Work out the finished part from the listing and answer in its coordinate system (mm). A direction names the side the tool comes from. Give positions to 0.01 mm unless a question says otherwise; leave off trailing zeros. Order: outer loops, then holes, each group sorted by start corner. A loop starts at its lowest first (then second) coordinate and runs counter-clockwise, first axis right, second up.
```python
from build123d import *

# Parameters (mm, degrees)
ESQUISSE1_R             = 75
ESQUISSE1_R_2           = 70
ESQUISSE1_R_3           = 2
ESQUISSE1_W             = 21
ESQUISSE1_H             = 41
BOSS_EXTRU_1_DEPTH      = 2
BOSS_EXTRU_2_START      = 40
ESQUISSE1_4_R           = 75
ESQUISSE1_4_R_2         = 70
BOSS_EXTRU_2_DEPTH      = 40
ESQUISSE2_W             = 20.133446777
ESQUISSE2_H             = 7.336961674
ENL_V_MAT_EXTRU_1_DEPTH = 40
ESQUISSE1_5_R           = 75
ESQUISSE1_5_R_2         = 70
BOSS_EXTRU_3_DEPTH      = 18


with BuildPart() as part:
    # Esquisse1 → Boss.-Extru.1 (new body)
    # profile 1 of 2: a face of its own
    with BuildSketch(Plane(origin=(0, 0, 0), x_dir=(1, 0, 0), z_dir=(0, 1, 0))):
        with Locations(Location((0, 0, 0), (0, 0, 270))):
            Circle(ESQUISSE1_R)
        Circle(ESQUISSE1_R_2, mode=Mode.SUBTRACT)
    # profile 2 of 2: a face of its own
    with BuildSketch(Plane(origin=(0, 0, 0), x_dir=(1, 0, 0), z_dir=(0, 1, 0))):
        Circle(ESQUISSE1_R_2)
        with Locations(Location((5, 14.17927264, 0), (0, 0, 270))):
            Circle(ESQUISSE1_R_3, mode=Mode.SUBTRACT)
        with Locations(Location((-5, 14.17927264, 0), (0, 0, 270))):
            Circle(ESQUISSE1_R_3, mode=Mode.SUBTRACT)
        with Locations(Location((-5, -34.45072736, 0), (0, 0, 270))):
            Circle(ESQUISSE1_R_3, mode=Mode.SUBTRACT)
        with Locations(Location((5, -34.45072736, 0), (0, 0, 270))):
            Circle(ESQUISSE1_R_3, mode=Mode.SUBTRACT)
        with Locations((0, -10.2)):
            Rectangle(ESQUISSE1_W, ESQUISSE1_H, mode=Mode.SUBTRACT)
    extrude(amount=-BOSS_EXTRU_1_DEPTH)

    # Esquisse1_4 → Boss.-Extru.2 (add)
    with BuildSketch(Plane(origin=(0, 0, 0), x_dir=(1, 0, 0), z_dir=(0, 1, 0)).offset(BOSS_EXTRU_2_START)):
        with Locations(Location((0, 0, 0), (0, 0, 270))):
            Circle(ESQUISSE1_4_R)
        with Locations(Location((0, 0, 0), (0, 0, 270))):
            Circle(ESQUISSE1_4_R_2, mode=Mode.SUBTRACT)
    extrude(amount=-BOSS_EXTRU_2_DEPTH)

    # Esquisse2 → Enl_v. mat.-Extru.1 (cut)
    with BuildSketch(Plane.XY.offset(75)):
        with Locations((0.592594447, 36.707948234)):
            Rectangle(ESQUISSE2_W, ESQUISSE2_H)
    extrude(amount=-ENL_V_MAT_EXTRU_1_DEPTH, mode=Mode.SUBTRACT)

    # Esquisse1_5 → Boss.-Extru.3 (add)
    with BuildSketch(Plane(origin=(0, 0, 0), x_dir=(1, 0, 0), z_dir=(0, 1, 0))):
        with Locations(Location((0, 0, 0), (0, 0, 270))):
            Circle(ESQUISSE1_5_R)
        with Locations(Location((0, 0, 0), (0, 0, 278.758845406))):
            Circle(ESQUISSE1_5_R_2, mode=Mode.SUBTRACT)
    extrude(amount=-BOSS_EXTRU_3_DEPTH)


solid = part.part
```
1. The part is cut by section D-D (x = -37). Write down the section's boundary in (y, z), then the cut area to 3 significant figures.
Findings below:
outline: (-18, -65.24) - (40, -65.24) - (40, -59.42) - (0, -59.42) - (0, 59.42) - (40, 59.42) - (40, 65.24) - (-18, 65.24) - (-18, 59.42) - (-2, 59.42) - (-2, -59.42) - (-18, -59.42) - close
area: 912 mm2
2. Which of the six approach directions +Z, -Z, +X, -X, +Y, -Y give full straight-line access (tool end or side, diameter ignored) to faces 1 (the face through (-9.474, 36, 72)), 2 (the face through (-16.65, -9.89, 67.99)), 3 (the face through (-42.594, 20.28, -55.55)), 4 (the face through (-50, -18, 50))?
Findings below:
face 1: +Z, +Y
face 2: -Y
face 3: +Y
face 4: +Z, -Z, +X, -X, -Y
3. The part is cut by section B-B (x = 0). Write down the section's boundary in (y, z), then the cut area to 3 significant figures.
Findings below:
outline: (-18, -75) - (40, -75) - (40, -70) - (0, -70) - (0, -10.3) - (-2, -10.3) - (-2, -70) - (-18, -70) - close; (-18, 70) - (-2, 70) - (-2, 30.7) - (0, 30.7) - (0, 70) - (33.04, 70) - (33.04, 75) - (-18, 75) - close
area: 743 mm2
4. The part is cut by section C-C (y = 7.5). Write down the section's boundary in (x, z).
Findings below:
outline: circle Ø150 at (0, 0); hole circle Ø140 at (0, 0)
5. The part is cut by section A-A (z = 0). Write down the section's boundary in (x, y).
Findings below:
outline: (-75, -18) - (-70, -18) - (-70, -2) - (-10.5, -2) - (-10.5, 0) - (-70, 0) - (-70, 40) - (-75, 40) - close; (10.5, -2) - (70, -2) - (70, -18) - (75, -18) - (75, 40) - (70, 40) - (70, 0) - (10.5, 0) - close
6. Straight lines are drawn through the part: probe 1 along X at (y, z) = (11.5, 0); probe 2 along Y at (x, z) = (33, 37.5). For each, find the intervals that lie inside material, in ascending order.
Findings below:
probe 1: x = -75 to -70, 70 to 75
probe 2: y = -2 to 0
7. Given P1, Ø1.5, axis at x = 37, z = 49, coming from the +Y side; P2, Ø1.7, axis at x = -2, z = 72, coming from the +Y side; P3, Ø5, axis at y = 23, z = -12, coming from the -X side, each flat-ended and moving along its own axis, determine where each tip first touches the part or whether it passes through.
Findings below:
P1: stops at y = 0
P2: stops at y = 33.04
P3: stops at x = -74.4
